from build123d import *

# Parameters (mm, degrees)
SKETCH1_R           = 4.25
BOSS_EXTRUDE1_DEPTH = 5
SKETCH2_R           = 27.5
CUT_EXTRUDE1_DEPTH  = 1
CHAMFER1_SIZE       = 1


with BuildPart() as part:
    # Sketch1 → Boss-Extrude1 (new body)
    with BuildSketch(Plane(origin=(0, 0, 0), x_dir=(1, 0, 0), z_dir=(0, 1, 0))):
        with BuildLine():
            Line((55, 8.5), (28.770644762, 8.5))
            ThreePointArc((28.770644762, 8.5), (22.669615426, 19.649135769), (12.5, 27.271780287))
            Line((12.5, 27.271780287), (12.5, 0))
            ThreePointArc((12.5, 0), (0, -12.5), (-12.5, 0))
            Line((-12.5, 0), (-12.5, 27.271780287))
            ThreePointArc((-12.5, 27.271780287), (-22.669615426, 19.649135769), (-28.770644762, 8.5))
            Line((-28.770644762, 8.5), (-55, 8.5))
            ThreePointArc((-55, 8.5), (-63.5, 0), (-55, -8.5))
            Line((-55, -8.5), (-28.770644762, -8.5))
            ThreePointArc((-28.770644762, -8.5), (0, -30), (28.770644762, -8.5))
            Line((28.770644762, -8.5), (55, -8.5))
            ThreePointArc((55, -8.5), (63.5, 0), (55, 8.5))
        make_face()
        with Locations(Location((-55, 0, 0), (0, 0, 270))):
            Circle(SKETCH1_R, mode=Mode.SUBTRACT)
        with Locations(Location((55, 0, 0), (0, 0, 270))):
            Circle(SKETCH1_R, mode=Mode.SUBTRACT)
    extrude(amount=BOSS_EXTRUDE1_DEPTH)

    # Sketch2 → Cut-Extrude1 (cut)
    with BuildSketch(Plane(origin=(0, 0, 0), x_dir=(1, 0, 0), z_dir=(0, 1, 0))):
        Circle(SKETCH2_R)
    extrude(amount=CUT_EXTRUDE1_DEPTH, mode=Mode.SUBTRACT)

    # Chamfer1
    chamfer1_edges = [part.edges().sort_by_distance(p)[0] for p in [
        (0, 0, 27.5),
    ]]
    chamfer(chamfer1_edges, length=CHAMFER1_SIZE - 0.0001)  # a hair under: the kernel refuses the full size


solid = part.part
Part model, mm, in its own coordinate system. A direction names the side the tool comes from. Coordinates: 2 decimals unless noted, no trailing zeros. Loops run counter-clockwise (first coordinate to the right, second up) from the corner with the lowest first, then second, coordinate; pieces in that order, holes last. Notation, with made-up numbers: M -8,71 L 41,71 A28 cw 41,109 Z; hole C -5,77 d9. An arc over 180 degrees is marked long. Use a Markdown table: item, result. Add a question column.
Q1. Which spindle directions (+Z, -Z, +X, -X, +Y, -Y) get a long thin tool onto all of the face, cutting with end or side? Do faces 1 (the flat face through (12.5, 3, -14)), 2 (the flat face through (-42, 2, -8.5)), 3 (the flat face through (42, 2, 8.5)), 4 (the flat face through (0, 1, 13)). Say none if no direction does.
Q2. Cut at C-C (z = 1.5). Give the number of separate pieces and of enclosed holes in the cut face, and give its area (3 significant figures).
Q3. Mould opens along Z. For faces 5 (the flat face through (-29, 0, -1)), 6 (the cylindrical face through (-59.15, 2.46, -0.92)), 7 (the flat face through (42, 2, -8.5)), 8 (the flat face through (-42, 2, 8.5)) say: +Z half, -Z half, draft (parallel to the pull), parting line (faces both ways), or undercut.
Q4. Pin check, flat tips, straight feed: P1, Ø2.5, axis at y = 2.5, z = -10.5, coming from the +X side; P2, Ø3, axis at x = 17.5, y = 3, coming from the -Z side; P3, Ø2.5, axis at x = -47, y = 2, coming from the +Z side. Stop position of each tip, or through.
Q5. Cut at D-D (x = 46). Write the cut outline in (y, z).
Q6. Probe L1, parallel to Z at x = -36.5, y = 1.75; L2, parallel to Y at x = 9.5, z = 20; L3, parallel to Z at x = 0, y = 1.05. List the from-to ranges inside material, lowest first.
Q7. Cut at A-A (y = 3.25). Write the cut outline in (x, z).
Worked out:
| question | item | result |
|---|---|---|
| 1 | face 1 | -Z, +Y, -Y |
| 1 | face 2 | -Z, -X, +Y, -Y |
| 1 | face 3 | +Z, +X, +Y, -Y |
| 1 | face 4 | -Y |
| 2 | separate pieces | 4 |
| 2 | enclosed holes | 0 |
| 2 | area | 399 mm2 |
| 3 | face 5 | draft |
| 3 | face 6 | undercut |
| 3 | face 7 | -Z half |
| 3 | face 8 | +Z half |
| 4 | P1 | stops at x = 28.54 |
| 4 | P2 | stops at z = -25.38 |
| 4 | P3 | stops at z = 8.5 |
| 5 | outline | M 0,-8.5 L 5,-8.5 L 5,8.5 L 0,8.5 Z |
| 6 | L1 | z = -8.5 to 8.5 |
| 6 | L2 | y = 1 to 5 |
| 6 | L3 | z = 12.5 to 30 |
| 7 | outline | M -55,-8.5 L -28.77,-8.5 A30 ccw -12.5,-27.27 L -12.5,0 A12.5 cw 12.5,0 L 12.5,-27.27 A30 ccw 28.77,-8.5 L 55,-8.5 A8.5 ccw 55,8.5 L 28.77,8.5 A30 ccw -28.77,8.5 L -55,8.5 A8.5 ccw Z; hole C -55,0 d8.5; hole C 55,0 d8.5 |
